For this review, take the finished solid that the model builds, in its own axes (mm). Round coordinates to 2 decimals unless told otherwise and drop trailing zeros. Write each loop counter-clockwise with the first axis right and the second up, starting at its lowest first coordinate (ties: lowest second). Pieces come first, ordered by that corner, then holes. Notation, with made-up numbers: (48, -12) -> (53, -12) arc R14 ccw to (53, 8) -> close; hole circle Ø8 at (66, 56). An arc over 180 degrees is marked (long way). Answer in a Markdown table with one row per item.
from build123d import *

# Parameters (mm, degrees)
SKETCH1_W           = 29
SKETCH1_H           = 110
BOSS_EXTRUDE1_DEPTH = 5
SKETCH2_R           = 2.413
CUT_EXTRUDE5_DEPTH  = 58.098598932
SKETCH3_W           = 12
SKETCH3_H           = 70
CUT_EXTRUDE6_DEPTH  = 1.5


with BuildPart() as part:
    # Sketch1 → Boss-Extrude1 (new body)
    with BuildSketch(Plane(origin=(0, 0, 0), x_dir=(1, 0, 0), z_dir=(0, 1, 0))):
        Rectangle(SKETCH1_W, SKETCH1_H)
    extrude(amount=BOSS_EXTRUDE1_DEPTH)

    # Sketch2 → Cut-Extrude5 (cut, through all)
    with BuildSketch(Plane(origin=(0, 5, 0), x_dir=(1, 0, 0), z_dir=(0, 1, 0))):
        with Locations(Location((-9, 45, 0), (0, 0, 270))):
            Circle(SKETCH2_R)
        with Locations(Location((9, 45, 0), (0, 0, 270))):
            Circle(SKETCH2_R)
        with Locations(Location((9, -45, 0), (0, 0, 270))):
            Circle(SKETCH2_R)
        with Locations(Location((-9, -45, 0), (0, 0, 270))):
            Circle(SKETCH2_R)
    extrude(amount=-CUT_EXTRUDE5_DEPTH, mode=Mode.SUBTRACT)

    # Sketch3 → Cut-Extrude6 (cut)
    with BuildSketch(Plane(origin=(0, 5, 0), x_dir=(1, 0, 0), z_dir=(0, 1, 0))):
        Rectangle(SKETCH3_W, SKETCH3_H)
    extrude(amount=-CUT_EXTRUDE6_DEPTH, mode=Mode.SUBTRACT)


solid = part.part
1) Consider section B-B on y = 1.65. State the section outline as (x, z) points, then the cut area to 3 significant figures.
Solved:
| item | result |
|---|---|
| outline | (-14.5, -55) -> (14.5, -55) -> (14.5, 55) -> (-14.5, 55) -> close; hole circle Ø4.83 at (-9, -45); hole circle Ø4.83 at (-9, 45); hole circle Ø4.83 at (9, -45); hole circle Ø4.83 at (9, 45) |
| area | 3,120 mm² |
2) Mouldability with a two-part tool opening along X and no side actions: class faces 1 (the flat face through (0, 3.5, 0)), 2 (the flat face through (-14.5, 2, 1)), 3 (the flat face through (0, 0, -1)) as pulls with the +X half, pulls with the -X half, needs draft (parallel to the pull), parting line crosses it, or undercut.
Solved:
| item | result |
|---|---|
| face 1 | undercut |
| face 2 | pulls with the -X half |
| face 3 | needs draft |
3) Consider section A-A on z = -45. State the section outline as (x, y) points, then the cut area to 3 significant figures.
Solved:
| item | result |
|---|---|
| outline | (-14.5, 0) -> (-11.41, 0) -> (-11.41, 5) -> (-14.5, 5) -> close; (-6.59, 0) -> (6.59, 0) -> (6.59, 5) -> (-6.59, 5) -> close; (11.41, 0) -> (14.5, 0) -> (14.5, 5) -> (11.41, 5) -> close |
| area | 96.7 mm² |
4) Consider section C-C on x = -9. State the section outline as (y, z) points, then the cut area to 3 significant figures.
Solved:
| item | result |
|---|---|
| outline | (0, -55) -> (5, -55) -> (5, -47.41) -> (0, -47.41) -> close; (0, -42.59) -> (5, -42.59) -> (5, 42.59) -> (0, 42.59) -> close; (0, 47.41) -> (5, 47.41) -> (5, 55) -> (0, 55) -> close |
| area | 502 mm² |
5) Consider section D-D on x = 2. State the section outline as (y, z) points, then the cut area to 3 significant figures.
Solved:
| item | result |
|---|---|
| outline | (0, -55) -> (5, -55) -> (5, -35) -> (3.5, -35) -> (3.5, 35) -> (5, 35) -> (5, 55) -> (0, 55) -> close |
| area | 445 mm² |
6) Clearance check with a flat-ended pin moving along its axis: pin 1 Ø3 at (x, z) = (-9, -45) entering from +Y. State where the tip first meets the part, or that it passes through.
Solved:
| item | result |
|---|---|
| pin 1 | through |
7) For line 1 (X direction, y = 2.6, z = -45); line 2 (Z direction, x = 9.5, y = 3.3); line 3 (Z direction, x = 7.25, y = 1), list the stretches that pass through material, from the lowest coordinate up. Write a range as [from, to].
Solved:
| item | result |
|---|---|
| line 1 | [-14.5, -11.41], [-6.59, 6.59], [11.41, 14.5] |
| line 2 | [-55, -47.36], [-42.64, 42.64], [47.36, 55] |
| line 3 | [-55, -46.66], [-43.34, 43.34], [46.66, 55] |
